Could you check a few things on this model? Use its own coordinates, in mm. A direction names the side the tool comes from. Coordinates: 2 decimals unless noted, no trailing zeros. Write each loop counter-clockwise with the first axis right and the second up, starting at its lowest first coordinate (ties: lowest second). Pieces come first, ordered by that corner, then holes.
Item 1: For P1, Ø8, axis at x = 19.5, y = 15, coming from the +Z side, with a flat end and sliding along its axis, tell me the tip position at first contact or that it passes through.
Item 2: I want a section at D-D on z = -1.1. State how many separate pieces and enclosed holes the cut face has, then the cut area to 3 significant figures.
Item 3: Thinking about a two-plate mould opening in X: for faces 1 (the flat face through (-9, 19, -1.75)), 2 (the cylindrical face through (-1, 24.73, -0.86)), 3 (the cylindrical face through (-7.15, -16.9, -0.86)), which applies, +X half, -X half, draft (parallel to the pull), parting line (faces both ways), or undercut?
Item 4: I want a section at C-C on x = 18. Please give me the cut outline in (y, z), then the cut area to 3 significant figures.
Item 5: If I drill on probe 1 along Y at (x, z) = (9, -0.7); probe 2 along Y at (x, z) = (6.5, -0.4); probe 3 along Y at (x, z) = (-15.5, -0.9), over which ranges is the centre line in solid material (lowest first)?
Item 6: I want a section at A-A on x = 8. Please give me the cut outline in (y, z), then the cut area to 3 significant figures.
Item 7: Which directions (+Z, -Z, +X, -X, +Y, -Y) give clear straight access to the entire face, cutting with the end or side of a thin tool? Please do faces 4 (the flat face through (-9, 19, 0)), 5 (the cylindrical face through (7.15, -16.9, -0.86)).
Item 8: I want a section at B-B on y = -10.5. Please give me the cut outline in (x, z).
from build123d import *

# Parameters (mm, degrees)
BODYSKE_R    = 1.25
BODY_DEPTH   = 1.75
MODLUGSKE_R  = 1.25
MODLUG_DEPTH = 1.75


with BuildPart() as part:
    # BodySke → Body (new body)
    with BuildSketch(Plane.XY):
        with BuildLine():
            Line((6.436111652, -23.898513904), (5.400081715, -20.051536536))
            ThreePointArc((5.400081715, -20.051536536), (6.699668105, -17.096735495), (9.864304114, -17.733016019))
            ThreePointArc((9.864304114, -17.733016019), (11.581275555, -18.645865936), (13.446997724, -18.097808741))
            ThreePointArc((13.446997724, -18.097808741), (0, 20.35), (-13.446997724, -18.097808741))
            ThreePointArc((-13.446997724, -18.097808741), (-11.581275555, -18.645865936), (-9.864304114, -17.733016019))
            ThreePointArc((-9.864304114, -17.733016019), (-6.699668105, -17.096735495), (-5.400081715, -20.051536536))
            Line((-5.400081715, -20.051536536), (-6.436111652, -23.898513904))
            ThreePointArc((-6.436111652, -23.898513904), (0, 24.75), (6.436111652, -23.898513904))
        make_face()
        with Locations((7.886492758, -19.38192088)):
            Circle(BODYSKE_R, mode=Mode.SUBTRACT)
        with Locations((-7.886492758, -19.38192088)):
            Circle(BODYSKE_R, mode=Mode.SUBTRACT)
    extrude(amount=-BODY_DEPTH)

    # ModLugSke → ModLug (add, through all)
    # profile 1 of 2: a face of its own
    with BuildSketch(Plane.XY):
        with BuildLine():
            Line((6.436111652, -23.898513904), (4.797758213, -17.814994138))
            ThreePointArc((4.797758213, -17.814994138), (4.807517042, -17.739334665), (4.867790397, -17.692572358))
            ThreePointArc((4.867790397, -17.692572358), (7.17874809, -16.887512424), (9.362030953, -15.78210621))
            ThreePointArc((9.362030953, -15.78210621), (9.431060859, -15.76974753), (9.491233364, -15.805763285))
            ThreePointArc((9.491233364, -15.805763285), (12.415098782, -17.336547673), (15.517305658, -16.210225194))
            Line((15.517305658, -16.210225194), (17.114597599, -17.878843615))
            ThreePointArc((17.114597599, -17.878843615), (12.153932868, -21.56025083), (6.436111652, -23.898513904))
        make_face()
        with Locations((7.886492758, -19.38192088)):
            Circle(MODLUGSKE_R, mode=Mode.SUBTRACT)
    # profile 2 of 2: a face of its own
    with BuildSketch(Plane.XY):
        with BuildLine():
            Line((-6.436111652, -23.898513904), (-4.797758213, -17.814994138))
            ThreePointArc((-4.797758213, -17.814994138), (-4.807517042, -17.739334665), (-4.867790397, -17.692572358))
            ThreePointArc((-4.867790397, -17.692572358), (-7.17874809, -16.887512424), (-9.362030953, -15.78210621))
            ThreePointArc((-9.362030953, -15.78210621), (-9.431060859, -15.76974753), (-9.491233364, -15.805763285))
            ThreePointArc((-9.491233364, -15.805763285), (-12.415098782, -17.336547673), (-15.517305658, -16.210225194))
            Line((-15.517305658, -16.210225194), (-17.114597599, -17.878843615))
            ThreePointArc((-17.114597599, -17.878843615), (-12.153932868, -21.56025083), (-6.436111652, -23.898513904))
        make_face()
        with Locations((-7.886492758, -19.38192088)):
            Circle(MODLUGSKE_R, mode=Mode.SUBTRACT)
    extrude(amount=-MODLUG_DEPTH)


solid = part.part
Response values:
1. P1: stops at z = 0
2. separate pieces: 1
2. enclosed holes: 2
2. area: 488 mm2
3. face 1: draft
3. face 2: parting line
3. face 3: undercut
4. outline: (-16.99, -1.75) - (-13.12, -1.75) - (-13.12, 0) - (-16.99, 0) - close; (10.67, -1.75) - (16.99, -1.75) - (16.99, 0) - (10.67, 0) - close
4. area: 17.8 mm2
5. probe 1: y = -23.06 to -19.95, -18.81 to -15.99, 18.38 to 23.06
5. probe 2: y = -23.88 to -17.16, 19.35 to 23.88
5. probe 3: y = -19.3 to -16.23, 13.78 to 19.3
6. outline: (-23.42, -1.75) - (-20.63, -1.75) - (-20.63, 0) - (-23.42, 0) - close; (-18.14, -1.75) - (-16.51, -1.75) - (-16.51, 0) - (-18.14, 0) - close; (18.81, -1.75) - (23.42, -1.75) - (23.42, 0) - (18.81, 0) - close
6. area: 15.8 mm2
7. face 4: +Z, +X, -X, +Y, -Y
7. face 5: +Z, -Z
8. outline: (-22.41, -1.75) - (-19.48, -1.75) - (-19.48, 0) - (-22.41, 0) - close; (19.48, -1.75) - (22.41, -1.75) - (22.41, 0) - (19.48, 0) - close
